Source: CAD feature listing. Evaluate the final solid. Frame: model axes, mm. A direction names the side the tool comes from. Round coordinates to 2 decimals unless told otherwise and drop trailing zeros. Order: outer loops, then holes, each group sorted by start corner. A loop starts at its lowest first (then second) coordinate and runs counter-clockwise, first axis right, second up. Notation, with made-up numbers: (77, 8) - (120, 8) arc R14 ccw to (120, 26) - close; hole circle Ø4 at (18.5, -23.75). An arc over 180 degrees is marked (long way). Return JSON: item names as keys, results as strings. Group by question number.
1) Section B-B, the plane y = 4.1. Give the number of separate pieces and of enclosed holes in the cut face, plus the area to 3 significant figures.
2) Mould query, pull axis X, two halves, no side actions, for faces 1 (the cylindrical face through (-85, 3, 54)), 2 (the cylindrical face through (-86.99, 2.54, -57.15)), 3 (the flat face through (90, 2, 1)). Classes: pulls with the +X half, pulls with the -X half, needs draft (parallel to the pull), parting line crosses it, or undercut.
3) Section A-A, the plane x = -58. Return loops of the section in (y, z), plus the area to 3 significant figures.
4) Contact query for flat-ended pins moving along their axis: P1, Ø1.6, axis at y = 3.5, z = 58, coming from the -X side; P2, Ø0.6, axis at y = 2, z = -58, coming from the +X side; P3, Ø0.6, axis at y = 2, z = 58.5, coming from the -X side. Output: stop coordinate, or through.
5) Section C-C, the plane x = 46. Return loops of the section in (y, z).
6) Ray query, line 1 (Z direction, x = 57, y = 1.6); line 2 (X direction, y = 4.5, z = 6.5); line 3 (Z direction, x = 4.5, y = 4.5). Return the intervals inside material, ascending. Write a range as from..to.
7) Section D-D, the plane z = 11.5. Return loops of the section in (x, y), plus the area to 3 significant figures.
8) Access query for faces 4 (the cylindrical face through (84, 3, -55)), 5 (the flat face through (-1, 2, 60)), 6 (the flat face through (55, 2, 59)). Directions: +Z, -Z, +X, -X, +Y, -Y. A direction counts if a zero-diameter tool reaches every point of the face in a straight line with its end or side. Return the directions, or none.
```python
from build123d import *

# Parameters (mm, degrees)
SKETCH1_W           = 180
SKETCH1_H           = 120
BOSS_EXTRUDE1_DEPTH = 5
FILLET1_R           = 10
FILLET2_R           = 10
FILLET3_R           = 10
FILLET4_R           = 10
SHELL1_T            = -4
SKETCH6_W           = 172
SKETCH6_H           = 112
CUT_EXTRUDE1_DEPTH  = 8.5
FILLET5_R           = 5
FILLET6_R           = 5
FILLET7_R           = 5
FILLET8_R           = 5
SKETCH8_W           = 10
SKETCH8_H           = 2
CUT_EXTRUDE2_DEPTH  = 8


with BuildPart() as part:
    # Sketch1 → Boss-Extrude1 (new body)
    with BuildSketch(Plane(origin=(0, 0, 0), x_dir=(1, 0, 0), z_dir=(0, 1, 0))):
        Rectangle(SKETCH1_W, SKETCH1_H)
    extrude(amount=BOSS_EXTRUDE1_DEPTH)

    # Fillet1
    fillet1_edges = [part.edges().sort_by_distance(p)[0] for p in [
        (-90, 2.5, 60),
    ]]
    fillet(fillet1_edges, radius=FILLET1_R)

    # Fillet2
    fillet2_edges = [part.edges().sort_by_distance(p)[0] for p in [
        (90, 2.5, 60),
    ]]
    fillet(fillet2_edges, radius=FILLET2_R)

    # Fillet3
    fillet3_edges = [part.edges().sort_by_distance(p)[0] for p in [
        (90, 2.5, -60),
    ]]
    fillet(fillet3_edges, radius=FILLET3_R)

    # Fillet4
    fillet4_edges = [part.edges().sort_by_distance(p)[0] for p in [
        (-90, 2.5, -60),
    ]]
    fillet(fillet4_edges, radius=FILLET4_R)

    # Shell1
    shell1_openings = [part.faces().sort_by_distance(p)[0] for p in [
        (0, 5, 0),
    ]]
    offset(amount=SHELL1_T, openings=shell1_openings, kind=Kind.INTERSECTION)

    # Sketch6 → Cut-Extrude1 (cut)
    with BuildSketch(Plane(origin=(0, 10, 0), x_dir=(1, 0, 0), z_dir=(0, 1, 0))):
        Rectangle(SKETCH6_W, SKETCH6_H)
    extrude(amount=-CUT_EXTRUDE1_DEPTH, mode=Mode.SUBTRACT)

    # Fillet5
    fillet5_edges = [part.edges().sort_by_distance(p)[0] for p in [
        (-86, 3.25, -56),
    ]]
    fillet(fillet5_edges, radius=FILLET5_R)

    # Fillet6
    fillet6_edges = [part.edges().sort_by_distance(p)[0] for p in [
        (86, 3.25, -56),
    ]]
    fillet(fillet6_edges, radius=FILLET6_R)

    # Fillet7
    fillet7_edges = [part.edges().sort_by_distance(p)[0] for p in [
        (-86, 3.25, 56),
    ]]
    fillet(fillet7_edges, radius=FILLET7_R)

    # Fillet8
    fillet8_edges = [part.edges().sort_by_distance(p)[0] for p in [
        (86, 3.25, 56),
    ]]
    fillet(fillet8_edges, radius=FILLET8_R)

    # Sketch8 → Cut-Extrude2 (cut)
    with BuildSketch(Plane(origin=(0, 0, 0), x_dir=(1, 0, 0), z_dir=(0, 1, 0))):
        with Locations((-55, 58)):
            Rectangle(SKETCH8_W, SKETCH8_H)
        with Locations((55, 58)):
            Rectangle(SKETCH8_W, SKETCH8_H)
        with Locations((55, -58)):
            Rectangle(SKETCH8_W, SKETCH8_H)
        with Locations((-55, -58)):
            Rectangle(SKETCH8_W, SKETCH8_H)
    extrude(amount=CUT_EXTRUDE2_DEPTH, mode=Mode.SUBTRACT)


solid = part.part
```
Geometry check:
{
 "1": {"separate pieces": "1", "enclosed holes": "5", "area": "2,190 mm2"},
 "2": {"face 1": "undercut", "face 2": "pulls with the -X half", "face 3": "pulls with the +X half"},
 "3": {"outline": "(0, -60) - (5, -60) - (5, -59) - (0, -59) - close; (0, -57) - (5, -57) - (5, -56) - (1.5, -56) - (1.5, 56) - (5, 56) - (5, 57) - (0, 57) - close; (0, 59) - (5, 59) - (5, 60) - (0, 60) - close", "area": "188 mm2"},
 "4": {"P1": "x = -86.94", "P2": "x = 86.38", "P3": "x = -85.72"},
 "5": {"outline": "(0, -60) - (5, -60) - (5, -56) - (1.5, -56) - (1.5, 56) - (5, 56) - (5, 60) - (0, 60) - close"},
 "6": {"line 1": "-60..-59, -57..-56, 56..57, 59..60", "line 2": "-90..-86, 86..90", "line 3": "-60..-56, 56..60"},
 "7": {"outline": "(-90, 0) - (90, 0) - (90, 5) - (86, 5) - (86, 1.5) - (-86, 1.5) - (-86, 5) - (-90, 5) - close", "area": "298 mm2"},
 "8": {"face 4": "+Y", "face 5": "+Z, +X, -X, +Y, -Y", "face 6": "+Y, -Y"}
}
